Can you work these out from the drawing? Everything is in mm from the part's minimum corner. A direction names the side the tool comes from. Coordinates: 2 decimals unless noted, no trailing zeros. Loops run counter-clockwise (first coordinate to the right, second up) from the corner with the lowest first, then second, coordinate; pieces in that order, holes last.
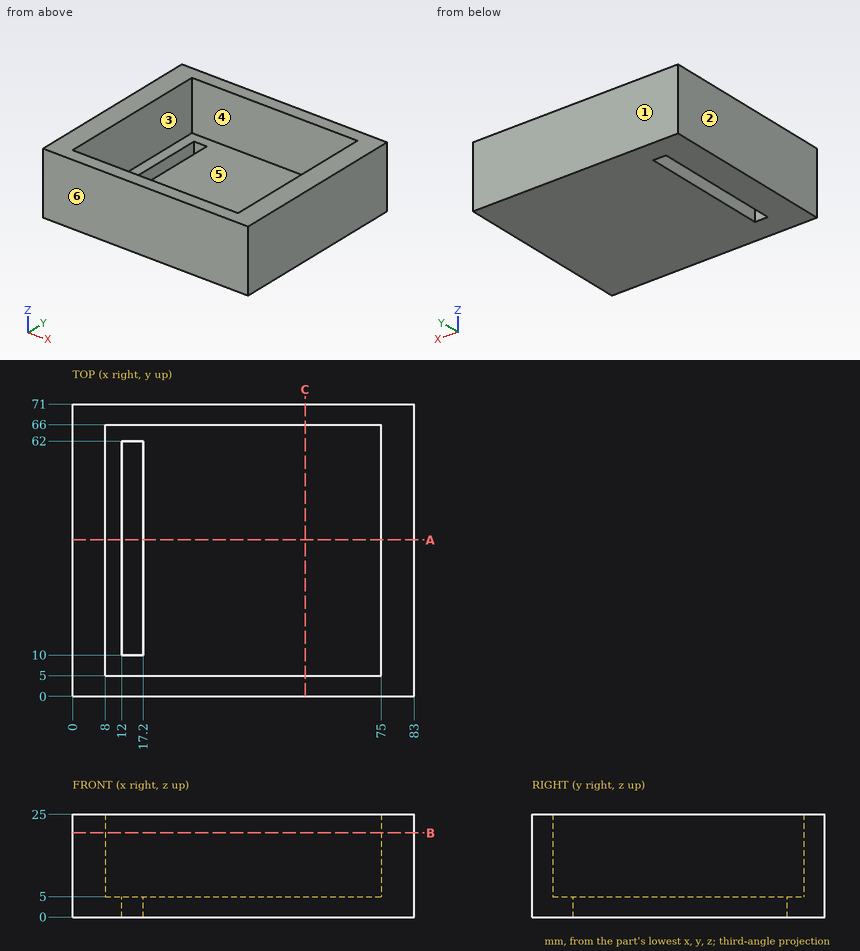
(1) Imagine slicing it at B-B, the plane z = 20.5. Write out the boundary of the cut face in (x, y).
Answers:
outline: (0, 0) - (83, 0) - (83, 71) - (0, 71) - close; hole (8, 5) - (75, 5) - (75, 66) - (8, 66) - close
(2) Imagine slicing it at C-C, the plane x = 56.5. Write out the boundary of the cut face in (y, z), and give its area (3 significant figures).
Answers:
outline: (0, 0) - (71, 0) - (71, 25) - (66, 25) - (66, 5) - (5, 5) - (5, 25) - (0, 25) - close
area: 555 mm2
(3) We'd pull the mould along X, two halves only. Please class the marked faces 1, 2, 3 and 4: +X half, -X half, draft (parallel to the pull), parting line (faces both ways), or undercut.
Answers:
face 1: draft
face 2: -X half
face 3: undercut
face 4: undercut
(4) For pin 1 (3 mm diameter, centred on x = 68, y = 57.5, fed in from +Z), with a flat end and sliding along its axis, tell me the tip position at first contact or that it passes through.
Answers:
pin 1: stops at z = 5
(5) I need wall thicknesses on probe 1 along Y at (x, z) = (53, 21.25); probe 2 along X at (y, z) = (18.5, 6.75); probe 3 along X at (y, z) = (47, 2.5). Which ranges of each line are inside material? Lowest first, please.
Answers:
probe 1: y = 0 to 5, 66 to 71
probe 2: x = 0 to 8, 75 to 83
probe 3: x = 0 to 12, 17.2 to 83
(6) Imagine slicing it at A-A, the plane y = 38. Write out the boundary of the cut face in (x, z), and give its area (3 significant figures).
Answers:
outline: (0, 0) - (12, 0) - (12, 5) - (8, 5) - (8, 25) - (0, 25) - close; (17.2, 0) - (83, 0) - (83, 25) - (75, 25) - (75, 5) - (17.2, 5) - close
area: 709 mm2
(7) Which directions (+Z, -Z, +X, -X, +Y, -Y) give clear straight access to the entire face, cutting with the end or side of a thin tool? Please do the marked faces 5 and 6.
Answers:
face 5: +Z
face 6: +Z, -Z, +X, -X, -Y
